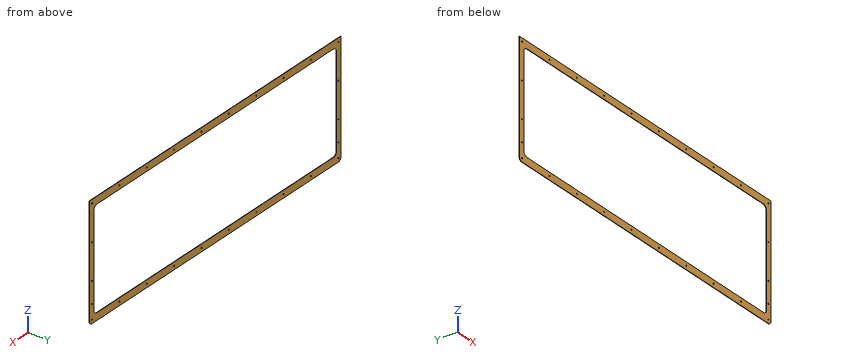
```python
from build123d import *

# Parameters (mm, degrees)
SZKIC4_R                    = 1.55
DODANIE_WYCI_GNI_CIE1_DEPTH = 1


with BuildPart() as part:
    # Szkic4 → Dodanie-wyciągnięcie1 (new body)
    with BuildSketch(Plane(origin=(0, 1505.947389818, 0), x_dir=(1, 0, 0), z_dir=(0, 1, 0))):
        with BuildLine():
            Line((11370.979687398, -709.37446721), (12194.979687398, -709.37446721))
            Line((12194.979687398, -709.37446721), (12194.979687398, -433.37446721))
            ThreePointArc((12194.979687398, -433.37446721), (12192.343648428, -427.010506179), (12185.979687398, -424.37446721))
            Line((12185.979687398, -424.37446721), (11379.979687398, -424.37446721))
            ThreePointArc((11379.979687398, -424.37446721), (11373.615726367, -427.010506179), (11370.979687398, -433.37446721))
            Line((11370.979687398, -433.37446721), (11370.979687398, -709.37446721))
        make_face()
        with Locations(Location((11379.979687398, -433.37446721, 0), (0, 0, 269.999999998))):
            Circle(SZKIC4_R, mode=Mode.SUBTRACT)
        with Locations(Location((11469.539687398, -433.37446721, 0), (0, 0, 269.999999998))):
            Circle(SZKIC4_R, mode=Mode.SUBTRACT)
        with Locations(Location((11559.094687398, -433.37446721, 0), (0, 0, 269.999999998))):
            Circle(SZKIC4_R, mode=Mode.SUBTRACT)
        with Locations(Location((11648.649687398, -433.37446721, 0), (0, 0, 269.999999998))):
            Circle(SZKIC4_R, mode=Mode.SUBTRACT)
        with Locations(Location((11738.204687398, -433.37446721, 0), (0, 0, 269.999999998))):
            Circle(SZKIC4_R, mode=Mode.SUBTRACT)
        with Locations(Location((11827.759687398, -433.37446721, 0), (0, 0, 269.999999998))):
            Circle(SZKIC4_R, mode=Mode.SUBTRACT)
        with Locations(Location((11917.314687398, -433.37446721, 0), (0, 0, 269.999999998))):
            Circle(SZKIC4_R, mode=Mode.SUBTRACT)
        with Locations(Location((12006.869687398, -433.37446721, 0), (0, 0, 269.999999998))):
            Circle(SZKIC4_R, mode=Mode.SUBTRACT)
        with Locations(Location((12096.424687398, -433.37446721, 0), (0, 0, 269.999999998))):
            Circle(SZKIC4_R, mode=Mode.SUBTRACT)
        with Locations(Location((12185.979687398, -433.37446721, 0), (0, 0, 269.999999998))):
            Circle(SZKIC4_R, mode=Mode.SUBTRACT)
        with Locations(Location((12185.979687398, -469.37446721, 0), (0, 0, 269.999999998))):
            Circle(SZKIC4_R, mode=Mode.SUBTRACT)
        with Locations(Location((12185.979687398, -522.37446721, 0), (0, 0, 269.999999998))):
            Circle(SZKIC4_R, mode=Mode.SUBTRACT)
        with Locations(Location((12185.979687398, -611.37446721, 0), (0, 0, 269.999999998))):
            Circle(SZKIC4_R, mode=Mode.SUBTRACT)
        with Locations(Location((12185.979687398, -700.37446721, 0), (0, 0, 269.999999998))):
            Circle(SZKIC4_R, mode=Mode.SUBTRACT)
        with Locations(Location((12096.419687398, -700.37446721, 0), (0, 0, 269.999999998))):
            Circle(SZKIC4_R, mode=Mode.SUBTRACT)
        with Locations(Location((12006.864687398, -700.37446721, 0), (0, 0, 269.999999998))):
            Circle(SZKIC4_R, mode=Mode.SUBTRACT)
        with Locations(Location((11917.309687398, -700.37446721, 0), (0, 0, 269.999999998))):
            Circle(SZKIC4_R, mode=Mode.SUBTRACT)
        with Locations(Location((11827.754687398, -700.37446721, 0), (0, 0, 269.999999998))):
            Circle(SZKIC4_R, mode=Mode.SUBTRACT)
        with Locations(Location((11738.199687398, -700.37446721, 0), (0, 0, 269.999999998))):
            Circle(SZKIC4_R, mode=Mode.SUBTRACT)
        with Locations(Location((11648.644687398, -700.37446721, 0), (0, 0, 269.999999998))):
            Circle(SZKIC4_R, mode=Mode.SUBTRACT)
        with Locations(Location((11559.089687398, -700.37446721, 0), (0, 0, 269.999999998))):
            Circle(SZKIC4_R, mode=Mode.SUBTRACT)
        with Locations(Location((11469.534687398, -700.37446721, 0), (0, 0, 269.999999998))):
            Circle(SZKIC4_R, mode=Mode.SUBTRACT)
        with Locations(Location((11379.979687398, -700.37446721, 0), (0, 0, 269.999999998))):
            Circle(SZKIC4_R, mode=Mode.SUBTRACT)
        with Locations(Location((11379.979687398, -611.37446721, 0), (0, 0, 269.999999998))):
            Circle(SZKIC4_R, mode=Mode.SUBTRACT)
        with Locations(Location((11379.979687398, -522.37446721, 0), (0, 0, 269.999999998))):
            Circle(SZKIC4_R, mode=Mode.SUBTRACT)
        with Locations(Location((11379.979687398, -469.37446721, 0), (0, 0, 269.999999998))):
            Circle(SZKIC4_R, mode=Mode.SUBTRACT)
        with BuildLine():
            Line((11385.979687398, -452.37446721), (11385.979687398, -680.37446721))
            ThreePointArc((11385.979687398, -680.37446721), (11389.201512805, -688.152641803), (11396.979687398, -691.37446721))
            Line((11396.979687398, -691.37446721), (12168.979687398, -691.37446721))
            ThreePointArc((12168.979687398, -691.37446721), (12176.757861991, -688.152641803), (12179.979687398, -680.37446721))
            Line((12179.979687398, -680.37446721), (12179.979687398, -452.37446721))
            ThreePointArc((12179.979687398, -452.37446721), (12177.05075521, -445.303399398), (12169.979687398, -442.37446721))
            Line((12169.979687398, -442.37446721), (11395.979687398, -442.37446721))
            ThreePointArc((11395.979687398, -442.37446721), (11388.908619586, -445.303399398), (11385.979687398, -452.37446721))
        make_face(mode=Mode.SUBTRACT)
    extrude(amount=DODANIE_WYCI_GNI_CIE1_DEPTH)


solid = part.part
```
Here's how the part is built. I have some questions about the finished solid (model axes, mm). Coordinates: 2 decimals unless noted, no trailing zeros. Write each loop counter-clockwise with the first axis right and the second up, starting at its lowest first coordinate (ties: lowest second). Pieces come first, ordered by that corner, then holes. Notation, with made-up numbers: (-3.75, 88.5) -> (44.25, 88.5) arc R11 cw to (44.25, 101.5) -> close; hole circle Ø10 at (-35, 30). An arc over 180 degrees is marked (long way). Use a Markdown table: item, result. Add a question column.
(1) If we section it at C-C, the plane y = 1506.1: State how many separate pieces and enclosed holes the cut face has, and give its area (3 significant figures).
(2) Please list where these lines run through material, in increasing order: line 1 (X direction, y = 1506.1, z = 612); line 2 (X direction, y = 1506.2, z = 492); line 3 (Z direction, x = 11460, y = 1506.15).
(3) If we section it at B-B, the plane x = 11675: Write out the boundary of the cut face in (y, z), and give its area (3 significant figures).
(4) If we section it at A-A, the plane z = 506: Write out the boundary of the cut face in (x, y), and give its area (3 significant figures).
Outcome:
| question | item | result |
|---|---|---|
| 1 | separate pieces | 1 |
| 1 | enclosed holes | 27 |
| 1 | area | 37,000 mm^2 |
| 2 | line 1 | x = 11370.98 to 11378.56, 11381.4 to 11385.98, 12179.98 to 12184.56, 12187.4 to 12194.98 |
| 2 | line 2 | x = 11370.98 to 11385.98, 12179.98 to 12194.98 |
| 2 | line 3 | z = 424.37 to 442.37, 691.37 to 709.37 |
| 3 | outline | (1505.95, 424.37) -> (1506.95, 424.37) -> (1506.95, 442.37) -> (1505.95, 442.37) -> close; (1505.95, 691.37) -> (1506.95, 691.37) -> (1506.95, 709.37) -> (1505.95, 709.37) -> close |
| 3 | area | 36.0 mm^2 |
| 4 | outline | (11370.98, 1505.95) -> (11385.98, 1505.95) -> (11385.98, 1506.95) -> (11370.98, 1506.95) -> close; (12179.98, 1505.95) -> (12194.98, 1505.95) -> (12194.98, 1506.95) -> (12179.98, 1506.95) -> close |
| 4 | area | 30.0 mm^2 |
